The model under review builds one solid part; all positions refer to its coordinate system, in mm. A direction names the side the tool comes from. Coordinates: 2 decimals unless noted, no trailing zeros. Order: outer loops, then holes, each group sorted by start corner. A loop starts at its lowest first (then second) coordinate and runs counter-clockwise, first axis right, second up.
Autodesk Inventor part; units mm, degrees
ref_plane "YZ Plane" through (0, 0, 0) normal (1, 0, 0) x (0, 1, 0)
ref_plane "XZ Plane" through (0, 0, 0) normal (0, 1, 0) x (-1, 0, 0)
ref_plane "XY Plane" through (0, 0, 0) normal (0, 0, 1) x (1, 0, 0)
sketch "Sketch1" plane through (0, 0, 0) normal (0, 1, 0) x (-1, 0, 0)
  line L0 (22.5526, 63.1659) -> (-40.8374, 63.1659)
  line L1 (-50.8374, 53.1659) -> (-50.8374, -18.3141)
  line L2 (-40.8374, -28.3141) -> (22.5526, -28.3141)
  line L3 (32.5526, -18.3141) -> (32.5526, 53.1659)
  arc A0 (32.5526, 53.1659) -> (22.5526, 63.1659) centre (22.5526, 53.1659) ccw
  arc A1 (22.5526, -28.3141) -> (32.5526, -18.3141) centre (22.5526, -18.3141) ccw
  arc A2 (-50.8374, -18.3141) -> (-40.8374, -28.3141) centre (-40.8374, -18.3141) ccw
  arc A3 (-40.8374, 63.1659) -> (-50.8374, 53.1659) centre (-40.8374, 53.1659) ccw
  point P0 (0, 0)
  point P1 (32.5526, 63.1659)
  point P2 (-50.8374, 63.1659)
  point P3 (32.5526, -28.3141)
  dimension "d0" = 83.39
  dimension "d1" = 91.48
  dimension "d2" = 10
  dimension "d3" = 10
extrude "Extrusion1" add sketch "Sketch1" along normal blind 23.54
sketch "Sketch2" plane through (40.8374, 0, -28.3141) normal (0, 0, -1) x (-1, 0, 0)
  line L0 (7.595, 14.9788) -> (21.095, 14.9788)
  line L1 (21.095, 14.9788) -> (21.095, 8.3788)
  line L2 (21.095, 8.3788) -> (7.595, 8.3788)
  line L3 (7.595, 8.3788) -> (7.595, 14.9788)
  line L4 (42.295, 14.9788) -> (55.795, 14.9788)
  line L5 (55.795, 14.9788) -> (55.795, 8.3788)
  line L6 (55.795, 8.3788) -> (42.295, 8.3788)
  line L7 (42.295, 8.3788) -> (42.295, 14.9788)
  line L8 (73.39, 0) -> (73.39, 23.54)
  point P0 (40.8374, 0)
  dimension "d6" = 13.5
  dimension "d7" = 6.6
  dimension "d8" = 13.5
  dimension "d9" = 6.6
  dimension "d10" = 21.2
  dimension "d11" = 17.595
extrude "Extrusion2" cut sketch "Sketch2" against normal blind 5
sketch "Sketch3" plane through (40.8374, 0, -28.3141) normal (0, 0, -1) x (-1, 0, 0)
  circle A0 centre (31.695, 11.77) radius 3
  line L0 (0, 23.54) -> (63.39, 23.54)
  line L1 (-10, 0) -> (-10, 23.54)
  point P0 (40.8374, 0)
  dimension "d14" = 6
  dimension "d15" = 11.77
  dimension "d16" = 41.695
extrude "Extrusion3" cut sketch "Sketch3" against normal blind 2
sketch "Sketch4" plane through (-32.5526, 0, -18.3141) normal (-1, 0, 0) x (0, 0, 1)
  line L0 (0, 15.77) -> (9.2, 15.77)
  line L1 (9.2, 15.77) -> (9.2, 11.77)
  line L2 (9.2, 11.77) -> (0, 11.77)
  line L3 (0, 11.77) -> (0, 15.77)
  line L4 (0, 0) -> (0, 23.54)
  line L5 (71.48, 0) -> (0, 0)
  point P0 (18.3141, 0)
  dimension "d19" = 9.2
  dimension "d20" = 4
  dimension "d21" = 0
  dimension "d22" = 11.77
extrude "Extrusion4" cut sketch "Sketch4" against normal blind 3
sketch "Sketch5" plane through (50.8374, 0, 53.1659) normal (1, 0, 0) x (0, 0, -1)
  line L0 (71.48, 15.77) -> (71.48, 23.54)
  line L1 (71.48, 20.37) -> (60.68, 20.37)
  line L2 (60.68, 20.37) -> (60.68, 11.77)
  line L3 (60.68, 11.77) -> (71.48, 11.77)
  line L4 (71.48, 11.77) -> (71.48, 20.37)
  line L5 (71.48, 0) -> (0, 0)
  point P0 (53.1659, 0)
  dimension "d25" = 8.6
  dimension "d26" = 10.8
  dimension "d27" = 11.77
extrude "Extrusion5" cut sketch "Sketch5" against normal blind 2
equation "\"d8\" = d6"
equation "\"d9\" = d7"
equation "\"d11\" = -d6 + 0.5 * d0 - 0.5 * d10"
equation "\"d16\" = 0.5 * d0"
properties part number "Yoobao"
(1) Wall thickness on line 1 (X direction, y = 13.5, z = -15.5); line 2 (Z direction, x = -27, y = 10); line 3 (Z direction, x = 46, y = 7.5): over which ranges is each line inside the solid? List them lowest first.
(2) Consider section A-A (x = -11). Give the boundary of the cut face in (y, z).
(3) Tool access review of faces 1 (the face through (9.79, 8.84, -27.33)), 2 (the face through (10, 23.54, 18)), 3 (the face through (-31, 14, -18.314)), 4 (the face through (50, 11.77, -13)): name each direction out of +Z, -Z, +X, -X, +Y, -Y from which nothing blocks a thin tool from reaching the whole face with its end or side.
(4) Insertion check: pin 1 Ø0.9 at (x, y) = (-31.5, 13.5) entering from +Z; pin 2 Ø5.5 at (y, z) = (13, -24.5) entering from -X; pin 3 Ø0.6 at (x, y) = (50, 15.5) entering from -Z. Each pin has a flat end and moves straight along its axis. Give the tip position at first contact, or say it passes through.
(5) The part is to be moulded in two halves that separate along X. For faces 5 (the face through (10, 0, 18)), 6 (the face through (-8, 14.979, -26)), 7 (the face through (-32.553, 12, 17)), say which applies: +X half, -X half, draft (parallel to the pull), parting line (faces both ways), or undercut.
Findings:
1. line 1: x = -29.55 to 48.84
1. line 2: z = -27.27 to 62.12
1. line 3: z = -26.88 to 61.73
2. outline: (0, -28.31) - (8.38, -28.31) - (8.38, -23.31) - (14.98, -23.31) - (14.98, -28.31) - (23.54, -28.31) - (23.54, 63.17) - (0, 63.17) - close
3. face 1: -Z
3. face 2: +Z, -Z, +X, -X, +Y
3. face 3: -X
3. face 4: +X
4. pin 1: stops at z = 58.44
4. pin 2: stops at x = -31.94
4. pin 3: stops at z = -22.95
5. face 5: draft
5. face 6: undercut
5. face 7: -X half
